For this review, use the dimensioned drawing (mm, ordinates from the lowest corner) and the shaded views. A direction names the side the tool comes from. Coordinates: 2 decimals unless noted, no trailing zeros. Write each loop counter-clockwise with the first axis right and the second up, starting at its lowest first coordinate (ties: lowest second). Pieces come first, ordered by that corner, then holes. Notation, with made-up numbers: (-26, 50) - (19, 50) arc R13 cw to (19, 63) - close; hole circle Ø2 at (6.25, 51.25). An arc over 180 degrees is marked (long way). Answer as a JSON object with one key per item and string values.
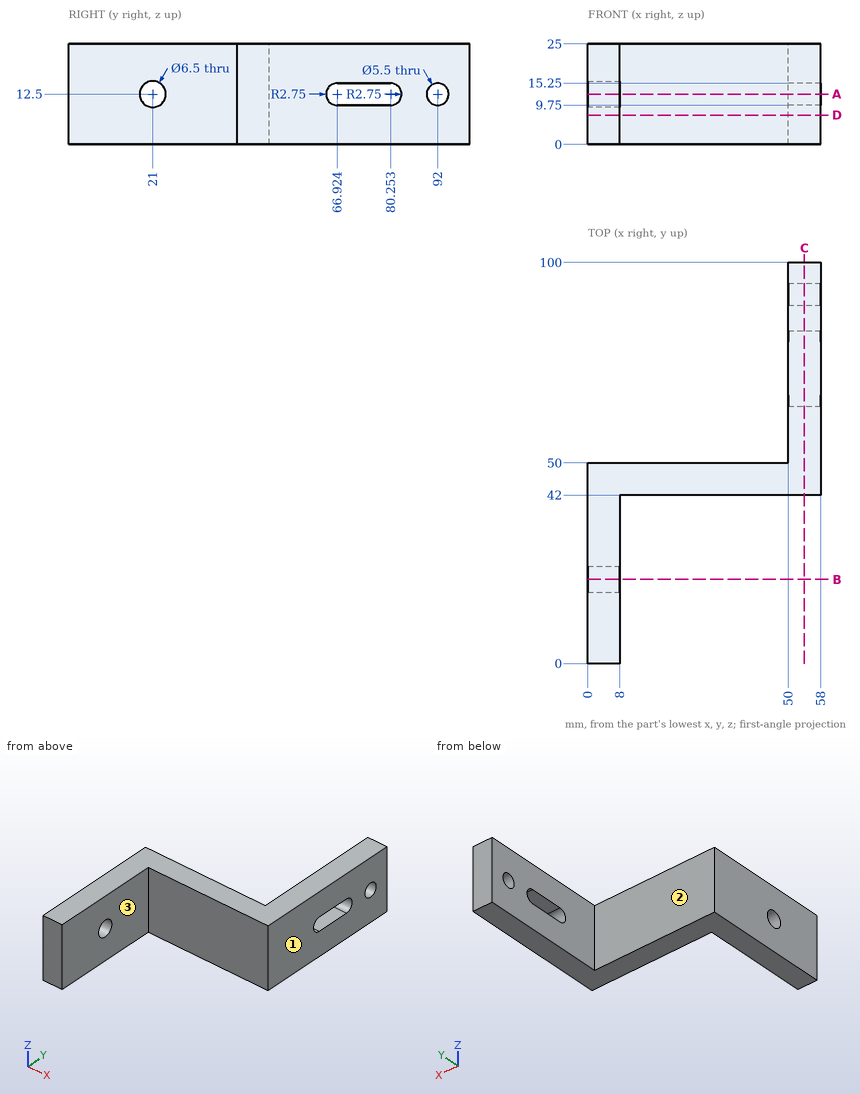
(1) Take a section at C-C, the plane x = 54. Write out the cut boundary in (y, z).
Solved:
{"outline": "(42, 0) - (100, 0) - (100, 25) - (42, 25) - close; hole (66.92, 9.75) - (80.25, 9.75) arc R2.75 ccw to (80.25, 15.25) - (66.92, 15.25) arc R2.75 ccw to start; hole circle Ø5.5 at (92, 12.5)"}
(2) Take a section at B-B, the plane y = 21. Write out the cut boundary in (x, z), and give its area (3 significant figures).
Solved:
{"outline": "(0, 0) - (8, 0) - (8, 9.25) - (0, 9.25) - close; (0, 15.75) - (8, 15.75) - (8, 25) - (0, 25) - close", "area": "148 mm^2"}
(3) For pin 1 (12.5 mm diameter, centred on x = 39.5, z = 15, fed in from -Y); pin 2 (10 mm diameter, centred on y = 65, z = 12.5, fed in from -X); pin 3 (9 mm diameter, centred on x = 52.5, y = 71.5, fed in from -Z); pin 4 (7.5 mm diameter, centred on y = 21, z = 12.5, fed in from +X), all flat-tipped, find the tip position at first contact; note any pin that passes through.
Solved:
{"pin 1": "stops at y = 42", "pin 2": "stops at x = 50", "pin 3": "stops at z = 0", "pin 4": "stops at x = 8"}
(4) Tool access review of the marked faces 1, 2 and 3: name each direction out of +Z, -Z, +X, -X, +Y, -Y from which nothing blocks a thin tool from reaching the whole face with its end or side.
Solved:
{"face 1": "+Z, -Z, +X, +Y, -Y", "face 2": "+Z, -Z, -X, +Y", "face 3": "+Z, -Z, +X, -Y"}
(5) Take a section at D-D, the plane z = 7.25. Write out the cut boundary in (x, y), and give its area (3 significant figures).
Solved:
{"outline": "(0, 0) - (8, 0) - (8, 42) - (58, 42) - (58, 100) - (50, 100) - (50, 50) - (0, 50) - close", "area": "1,200 mm^2"}
(6) To check wall thickness, follow line 1 (Y direction, x = 55, z = 12.5); line 2 (Y direction, x = 2.5, z = 12.5); line 3 (X direction, y = 5, z = 10). State the ranges of each line that lie inside material, in increasing order. Write a range as from..to.
Solved:
{"line 1": "y = 42..64.17, 83..89.25, 94.75..100", "line 2": "y = 0..17.75, 24.25..50", "line 3": "x = 0..8"}
(7) Take a section at A-A, the plane z = 12.5. Write out the cut boundary in (x, y).
Solved:
{"outline": "(0, 0) - (8, 0) - (8, 17.75) - (0, 17.75) - close; (0, 24.25) - (8, 24.25) - (8, 42) - (58, 42) - (58, 64.17) - (50, 64.17) - (50, 50) - (0, 50) - close; (50, 83) - (58, 83) - (58, 89.25) - (50, 89.25) - close; (50, 94.75) - (58, 94.75) - (58, 100) - (50, 100) - close"}
